Part model, mm, in its own coordinate system. Face numbers are marked on the shaded views. A direction names the side the tool comes from. Give positions to 0.01 mm unless a question says otherwise; leave off trailing zeros. Write each loop counter-clockwise with the first axis right and the second up, starting at its lowest first coordinate (ties: lowest second). Pieces come first, ordered by that corner, then holes. Notation, with made-up numbers: (-3, 67) - (55, 67) arc R18 cw to (55, 71) - close; hole circle Ø7 at (25.25, 17). An arc over 180 degrees is marked (long way). Answer as a JSON object with one key per item and string values. Group by question number.
```python
from build123d import *

# Parameters (mm, degrees)
F1_DEPTH = 63.5
F2_W     = 38.1
F2_H     = 6.35
F3_DEPTH = 63.501
F4_W     = 31.75
F4_H     = 7.874
F5_DEPTH = 38.101
F4_R     = 14.2875
F4_R_2   = 6.7437
F6_DEPTH = 9.2456
F7_DEPTH = 38.101
F8_W     = 63.5
F8_H     = 12.7
F9_DEPTH = 12.7


with BuildPart() as f1:
    # F0 (on Front) → F1 (new body)
    with BuildSketch(Plane.XZ):
        Polygon((0, 12.7), (0, 0), (47.498, 0), (47.498, -11.579418), (50.8, -11.579418), (50.8, -25.4), (63.5, -25.4), (63.5, 12.7), (47.498, 12.7), align=None)
    extrude(amount=F1_DEPTH)

    # F2 (on face) → F3 (cut, through all)
    with BuildSketch(Plane.YZ.offset(63.5)):
        with Locations((-31.75, -22.225)):
            Rectangle(F2_W, F2_H)
    extrude(amount=-F3_DEPTH, mode=Mode.SUBTRACT)

    # F4 (on face) → F5 (cut, through all)
    with BuildSketch(Plane.XY.offset(12.7)):
        with Locations((31.623, -3.937)):
            Rectangle(F4_W, F4_H)
        with Locations((31.623, -59.563)):
            Rectangle(F4_W, F4_H)
    extrude(amount=-F5_DEPTH, mode=Mode.SUBTRACT)

    # F4 (on face) → F6 (cut)
    with BuildSketch(Plane.XY.offset(12.7)):
        with Locations((31.75, -31.75)):
            Circle(F4_R)
        with Locations((31.75, -31.75)):
            Circle(F4_R_2, mode=Mode.SUBTRACT)
    extrude(amount=-F6_DEPTH, mode=Mode.SUBTRACT)

    # F4 (on face) → F7 (cut, through all)
    with BuildSketch(Plane.XY.offset(12.7)):
        with Locations((31.75, -31.75)):
            Circle(F4_R_2)
    extrude(amount=-F7_DEPTH, mode=Mode.SUBTRACT)

    # F8 (on face) → F9 (join)
    with BuildSketch(Plane(origin=(0, 0, 0), x_dir=(0, -1, 0), z_dir=(-1, 0, 0))):
        with BuildLine():
            Line((0, 35.052), (0, 12.7))
            Line((0, 12.7), (63.5, 12.7))
            Line((63.5, 12.7), (63.5, 35.052))
            ThreePointArc((63.5, 35.052), (59.780256, 44.032256), (50.8, 47.752))
            Line((50.8, 47.752), (12.7, 47.752))
            ThreePointArc((12.7, 47.752), (3.719744, 44.032256), (0, 35.052))
        make_face()
        with BuildLine():
            Line((13.693089, 42.863124), (51.793089, 42.863124))
            ThreePointArc((51.793089, 42.863124), (58.674, 35.052), (51.793089, 27.240876))
            Line((51.793089, 27.240876), (13.693089, 27.240876))
            ThreePointArc((13.693089, 27.240876), (4.826, 35.052), (13.693089, 42.863124))
        make_face(mode=Mode.SUBTRACT)
        with Locations((31.75, 6.35)):
            Rectangle(F8_W, F8_H)
    extrude(amount=F9_DEPTH)


solid = f1.part
```
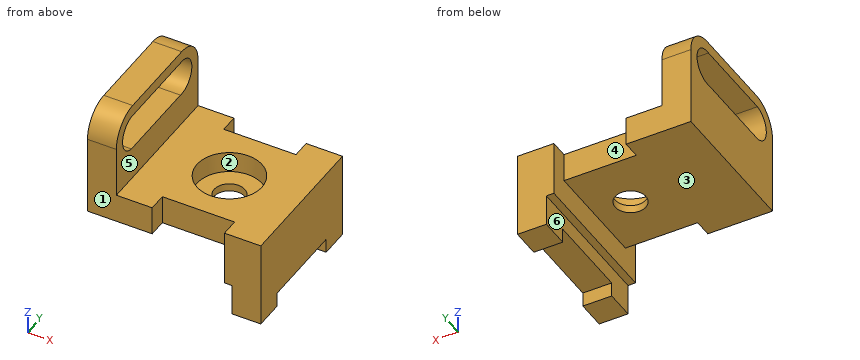
1) Band-saw the part on A-A (x = 31.75). List the corners of the cut face in (y, z), plus the area to 3 significant figures.
2) Band-saw the part on B-B (y = -31.75). List the corners of the cut face in (x, z), plus the area to 3 significant figures.
3) Drop flat-ended pins along their axis: P1, Ø6, axis at x = -4, y = -12.5, coming from the -Z side; P2, Ø3.5, axis at x = 49, y = -30.5, coming from the -Z side; P3, Ø7, axis at y = -32, z = -20.5, coming from the -X side; P4, Ø12, axis at x = 31.75, y = -31.75, coming from the +Z side. Give the stop position or say it passes through.
4) Mould opens along Y. For the marked faces 1, 2 and 3 say: pulls with the +Y half, pulls with the -Y half, needs draft (parallel to the pull), parting line crosses it, or undercut.
5) Probe line 1 (X direction, y = -31, z = 6); line 2 (Y direction, x = 31.75, z = 10.5); line 3 (Y direction, x = 31.75, z = 2.7). List the from-to ranges inside material, lowest first.
6) Band-saw the part on D-D (y = -9). List the corners of the cut face in (x, z), plus the area to 3 significant figures.
7) Band-saw the part on C-C (z = 37.5). List the corners of the cut face in (x, y).
8) Which spindle directions (+Z, -Z, +X, -X, +Y, -Y) get a long thin tool onto all of the face, cutting with end or side? Do the marked faces 4, 5 and 6. Say none if no direction does.
Verdict:
{
 "1": {"outline": "(-55.63, 0) - (-38.49, 0) - (-38.49, 3.45) - (-46.04, 3.45) - (-46.04, 12.7) - (-55.63, 12.7) - close; (-25.01, 0) - (-7.87, 0) - (-7.87, 12.7) - (-17.46, 12.7) - (-17.46, 3.45) - (-25.01, 3.45) - close", "area": "296 mm2"},
 "2": {"outline": "(-12.7, 0) - (25.01, 0) - (25.01, 3.45) - (17.46, 3.45) - (17.46, 12.7) - (0, 12.7) - (0, 27.24) - (-12.7, 27.24) - close; (-12.7, 42.86) - (0, 42.86) - (0, 47.75) - (-12.7, 47.75) - close; (38.49, 0) - (47.5, 0) - (47.5, -11.58) - (50.8, -11.58) - (50.8, -19.05) - (63.5, -19.05) - (63.5, 12.7) - (46.04, 12.7) - (46.04, 3.45) - (38.49, 3.45) - close", "area": "1,180 mm2"},
 "3": {"P1": "z = 0", "P2": "z = -11.58", "P3": "x = 50.8", "P4": "through"},
 "4": {"face 1": "pulls with the -Y half", "face 2": "undercut", "face 3": "needs draft"},
 "5": {"line 1": "-12.7 to 17.48, 46.02 to 63.5", "line 2": "-55.63 to -46.04, -17.46 to -7.87", "line 3": "-55.63 to -38.49, -25.01 to -7.87"},
 "6": {"outline": "(-12.7, 0) - (47.5, 0) - (47.5, -11.58) - (50.8, -11.58) - (50.8, -25.4) - (63.5, -25.4) - (63.5, 12.7) - (0, 12.7) - (0, 28.1) - (-12.7, 28.1) - close; (-12.7, 42) - (0, 42) - (0, 47.2) - (-12.7, 47.2) - close", "area": "1,590 mm2"},
 "7": {"outline": "(-12.7, -63.26) - (0, -63.26) - (0, -58.28) - (-12.7, -58.28) - close; (-12.7, -5.22) - (0, -5.22) - (0, -0.24) - (-12.7, -0.24) - close"},
 "8": {"face 4": "+Z, -Z, +Y", "face 5": "+Z, +X, +Y, -Y", "face 6": "-Z, -X, +Y, -Y"}
}
